Geometry check sheet. Reference: drawing and pictorial views, mm from the part's lowest x, y, z. A direction names the side the tool comes from. Give positions to 0.01 mm unless a question says otherwise; leave off trailing zeros. Write each loop counter-clockwise with the first axis right and the second up, starting at its lowest first coordinate (ties: lowest second). Pieces come first, ordered by that corner, then holes. Notation, with made-up numbers: (9.5, -31) - (35.5, -31) arc R26 ccw to (35.5, 7) - close; hole circle Ø4 at (-35.75, -14.75). An arc over 180 degrees is marked (long way). Put each result on its own line as item: value.
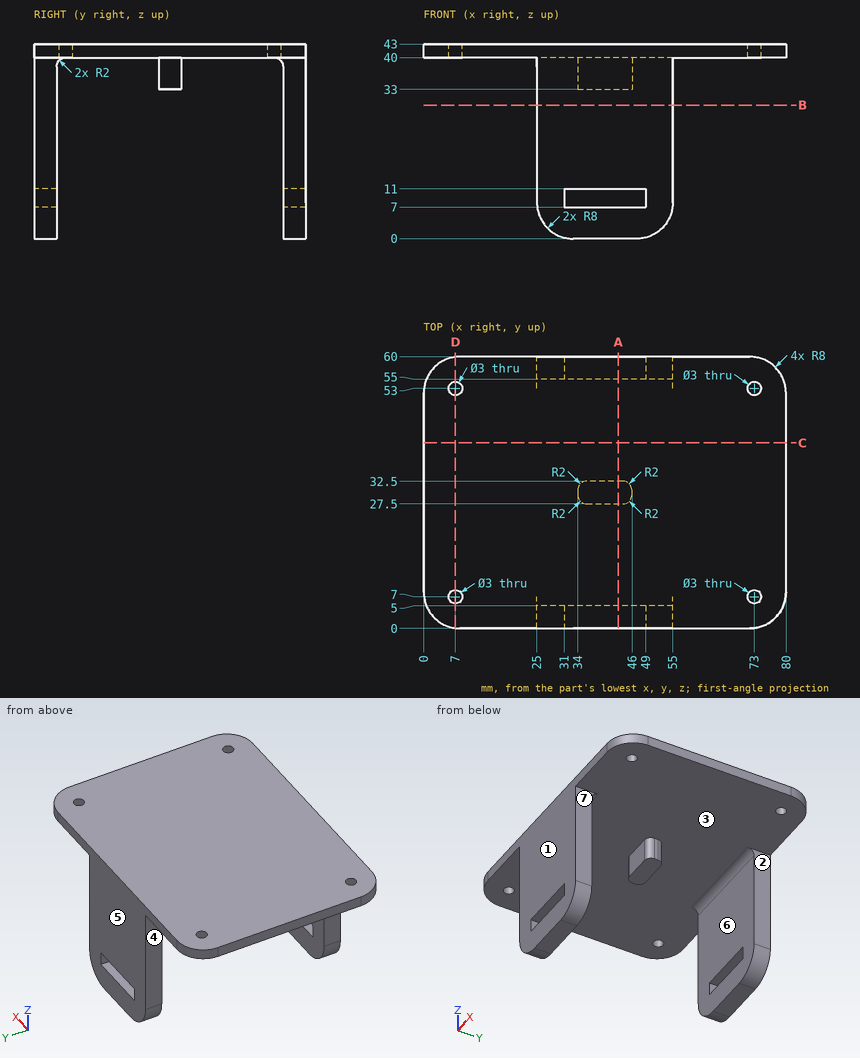
Q1. Section check A-A, the plane x = 43. Record the cut outline in (y, z), plus the area to 3 significant figures.
Answers follow:
outline: (0, 0) - (5, 0) - (5, 7) - (0, 7) - close; (0, 11) - (5, 11) - (5, 38) arc R2 cw to (7, 40) - (27.5, 40) - (27.5, 33) - (32.5, 33) - (32.5, 40) - (53, 40) arc R2 cw to (55, 38) - (55, 11) - (60, 11) - (60, 43) - (0, 43) - close; (55, 0) - (60, 0) - (60, 7) - (55, 7) - close
area: 577 mm2
Q2. Section check B-B, the plane z = 29.5. Record the cut outline in (x, y), plus the area to 3 significant figures.
Answers follow:
outline: (25, 0) - (55, 0) - (55, 5) - (25, 5) - close; (25, 55) - (55, 55) - (55, 60) - (25, 60) - close
area: 300 mm2
Q3. Section check D-D, the plane x = 7. Record the cut outline in (y, z), plus the area to 3 significant figures.
Answers follow:
outline: (0.06, 40) - (5.5, 40) - (5.5, 43) - (0.06, 43) - close; (8.5, 40) - (51.5, 40) - (51.5, 43) - (8.5, 43) - close; (54.5, 40) - (59.94, 40) - (59.94, 43) - (54.5, 43) - close
area: 162 mm2
Q4. Section check C-C, the plane y = 41. Record the cut outline in (x, z).
Answers follow:
outline: (0, 40) - (80, 40) - (80, 43) - (0, 43) - close
Q5. Go/stop test with flat-tipped pins: pin 1 Ø5.5 at (y, z) = (55, 24.5) entering from +X; pin 2 Ø4 at (x, y) = (73, 7) entering from -Z; pin 3 Ø1.8 at (x, y) = (7, 53) entering from +Z; pin 4 Ø1.2 at (y, z) = (2.5, 8) entering from -X. Record where each tip stops, or that it passes through.
Answers follow:
pin 1: stops at x = 55
pin 2: stops at z = 40
pin 3: passes through
pin 4: stops at x = 25
Q6. Set-up check for the marked faces 4, 5, 6 and 7: record each of +Z, -Z, +X, -X, +Y, -Y from which the full face is reachable in a straight line by a thin tool's end or side.
Answers follow:
face 4: -Z, -X, +Y, -Y
face 5: +Z, -Z, +X, -X, +Y
face 6: -Z, +X, -X
face 7: -Z, +X, +Y, -Y
Q7. Scan lines: line 1 along Y through (x, z) = (26.5, 30); line 2 along Y through (x, z) = (73, 40.7); line 3 along Z through (x, y) = (67, 35). Record each from-to range of solid material in increasing order.
Answers follow:
line 1: y = 0 to 5, 55 to 60
line 2: y = 0.06 to 5.5, 8.5 to 51.5, 54.5 to 59.94
line 3: z = 40 to 43
Q8. Release check for a two-part mould opening along Y. For the marked faces 1, 2 and 3 record: released by +Y, released by -Y, zero draft, split by the parting line, or undercut.
Answers follow:
face 1: released by -Y
face 2: zero draft
face 3: undercut
